Check sheet for the modelled part. Datum: model origin and axes. Units: mm. A direction names the side the tool comes from. Coordinates: 2 decimals unless noted, no trailing zeros. Loops run counter-clockwise (first coordinate to the right, second up) from the corner with the lowest first, then second, coordinate; pieces in that order, holes last. Notation, with made-up numbers: M 15.5,41 L 52.5,41 A9 ccw 52.5,46 Z; hole C 2,-29 d2. An arc over 180 degrees is marked long. Use CSV: the item, a comma, the result in double quotes. Start each with the question number.
(1) Section check D-D on z = 291. Record the cut outline in (x, y), and give its area (3 significant figures).
(2) Section check C-C on y = 0. Record the cut outline in (x, z).
(3) Section check A-A on x = -4. Record the cut outline in (y, z), and give its area (3 significant figures).
(4) Section check B-B on z = 450. Record the cut outline in (x, y), and give its area (3 significant figures).
(5) Scan lines: line 1 (Y direction, x = 10, z = 194.5); line 2 (Y direction, x = 15.5, z = 76.5). Record each from-to range of solid material in increasing order.
(6) Set-up check for faces 5 (the flat face through (-16, 0, 0)), 6 (the flat face through (0, 14.5, 246)): record each of +Z, -Z, +X, -X, +Y, -Y from which the full face is reachable in a straight line by a thin tool's end or side.
(7) Draft check along Y on faces 1 (the flat face through (-14.5, 0, 246)), 2 (the flat face through (0, 17.5, 246)), 3 (the flat face through (0, -14.5, 246)), 4 (the flat face through (0, -17.5, 246)). Enter one of: pulls with the +Y half, pulls with the -Y half, needs draft (parallel to the pull), parting line crosses it, or undercut.
from build123d import *

# Parameters (mm, degrees)
SZKIC1_W                    = 35
SZKIC1_H                    = 35
SZKIC1_W_2                  = 29
SZKIC1_H_2                  = 29
DODANIE_WYCI_GNI_CIE1_DEPTH = 500
WYTNIJ_WYCI_GNI_CIE1_REACH  = 503.529


with BuildPart() as part:
    # Szkic1 → Dodanie-wyciągnięcie1 (new body)
    with BuildSketch(Plane.XY):
        Rectangle(SZKIC1_W, SZKIC1_H)
        Rectangle(SZKIC1_W_2, SZKIC1_H_2, mode=Mode.SUBTRACT)
    extrude(amount=DODANIE_WYCI_GNI_CIE1_DEPTH)

    # Wytnij-wyciągnięcie1: up to this face of the body (flat: up to its plane)
    wytnij_wyci_gni_cie1_end = Plane(part.part.faces().sort_by_distance((-17.5, 0, 250))[0])
    # Szkic2 → Wytnij-wyciągnięcie1 (cut, up to the picked face)
    with BuildSketch(Plane(origin=(17.5, 0, 0), x_dir=(0, 0, -1), z_dir=(1, 0, 0)), mode=Mode.PRIVATE) as wytnij_wyci_gni_cie1_sk1:
        with BuildLine():
            Line((-455, 6), (-415, 6))
            ThreePointArc((-415, 6), (-409, 0), (-415, -6))
            Line((-415, -6), (-455, -6))
            ThreePointArc((-455, -6), (-461, 0), (-455, 6))
        make_face()
    wytnij_wyci_gni_cie1_tool1 = split(extrude(wytnij_wyci_gni_cie1_sk1.sketch, amount=-WYTNIJ_WYCI_GNI_CIE1_REACH, mode=Mode.PRIVATE), bisect_by=wytnij_wyci_gni_cie1_end, keep=Keep.BOTH, mode=Mode.PRIVATE)
    # Szkic2 → Wytnij-wyciągnięcie1 (cut, up to the picked face)
    with BuildSketch(Plane(origin=(17.5, 0, 0), x_dir=(0, 0, -1), z_dir=(1, 0, 0)), mode=Mode.PRIVATE) as wytnij_wyci_gni_cie1_sk2:
        with BuildLine():
            Line((-45, -6), (-85, -6))
            ThreePointArc((-85, -6), (-91, 0), (-85, 6))
            Line((-85, 6), (-45, 6))
            ThreePointArc((-45, 6), (-39, 0), (-45, -6))
        make_face()
    wytnij_wyci_gni_cie1_tool2 = split(extrude(wytnij_wyci_gni_cie1_sk2.sketch, amount=-WYTNIJ_WYCI_GNI_CIE1_REACH, mode=Mode.PRIVATE), bisect_by=wytnij_wyci_gni_cie1_end, keep=Keep.BOTH, mode=Mode.PRIVATE)
    add(wytnij_wyci_gni_cie1_tool1.solids().sort_by(Axis((17.5, 0, 435), (-1, 0, 0)))[0], mode=Mode.SUBTRACT)
    add(wytnij_wyci_gni_cie1_tool2.solids().sort_by(Axis((17.5, 0, 65), (-1, 0, 0)))[0], mode=Mode.SUBTRACT)


solid = part.part
Outcome:
1,outline,"M -17.5,-17.5 L 17.5,-17.5 L 17.5,17.5 L -17.5,17.5 Z; hole M -14.5,-14.5 L 14.5,-14.5 L 14.5,14.5 L -14.5,14.5 Z"
1,area,"384 mm²"
2,outline,"M -17.5,0 L -14.5,0 L -14.5,39 L -17.5,39 Z; M -17.5,91 L -14.5,91 L -14.5,409 L -17.5,409 Z; M -17.5,461 L -14.5,461 L -14.5,500 L -17.5,500 Z; M 14.5,0 L 17.5,0 L 17.5,39 L 14.5,39 Z; M 14.5,91 L 17.5,91 L 17.5,409 L 14.5,409 Z; M 14.5,461 L 17.5,461 L 17.5,500 L 14.5,500 Z"
3,outline,"M -17.5,0 L -14.5,0 L -14.5,500 L -17.5,500 Z; M 14.5,0 L 17.5,0 L 17.5,500 L 14.5,500 Z"
3,area,"3,000 mm²"
4,outline,"M -17.5,-17.5 L 17.5,-17.5 L 17.5,-6 L 14.5,-6 L 14.5,-14.5 L -14.5,-14.5 L -14.5,-6 L -17.5,-6 Z; M -17.5,6 L -14.5,6 L -14.5,14.5 L 14.5,14.5 L 14.5,6 L 17.5,6 L 17.5,17.5 L -17.5,17.5 Z"
4,area,"312 mm²"
5,line 1,"y = -17.5 to -14.5, 14.5 to 17.5"
5,line 2,"y = -17.5 to -6, 6 to 17.5"
6,face 5,"-Z, +X, -X, +Y, -Y"
6,face 6,"+Z, -Z"
7,face 1,"undercut"
7,face 2,"pulls with the +Y half"
7,face 3,"undercut"
7,face 4,"pulls with the -Y half"
